Can you work these out from the model? Positions are in its coordinate system, mm. A direction names the side the tool comes from. Round coordinates to 2 decimals unless told otherwise and drop trailing zeros. Order: outer loops, then holes, each group sorted by start corner. A loop starts at its lowest first (then second) coordinate and runs counter-clockwise, first axis right, second up.
Q1. If I drill on line 1 (Y direction, x = 13.75, z = 0.55); line 2 (Y direction, x = -9, z = 2.55); line 3 (Y direction, x = 13.75, z = 0.5), over which ranges is the centre line in solid material (lowest first)?
Q2. For faces 5 (the face through (-11.61, 17.9, 2.36)), 6 (the face through (-18.05, -3.64, 3.43)), 7 (the face through (13.3, 23, 0.5)), 8 (the face through (16, 17, 2)), which set-ups out of +Z, -Z, +X, -X, +Y, -Y let a thin tool reach every point of the face, with its end or its side?
Q3. If we section it at A-A (y = -17.5): Please give me the cut outline in (x, z) (3 decimals), plus the area to 3 significant figures.
Q4. Will these pins go through, and if not, where does the flat tip stop? P1, Ø3, axis at x = 11.5, y = 13, coming from the -Z side; P2, Ø1.9, axis at y = 22, z = 2, coming from the -X side; P3, Ø3, axis at x = -14.5, y = 20, coming from the +Z side; P4, Ø1.4, axis at x = 15.5, z = 2, coming from the +Y side.
Q5. We'd pull the mould along Y, two halves only. Please class faces 1 (the face through (0, 1, 0)), 2 (the face through (-13.2, 23, 0.5)), 3 (the face through (12.64, 21.01, 0.49)), 4 (the face through (-14.86, 21.01, 0.49)): pulls with the +Y half, pulls with the -Y half, needs draft (parallel to the pull), parting line crosses it, or undercut.
from build123d import *

# Parameters (mm, degrees)
RESSALTO_EXTRUS_O1_DEPTH = 3.75
ESBO_O1_3_R              = 1.5
RESSALTO_EXTRUS_O2_DEPTH = 1
CORTE_EXTRUS_O1_DEPTH    = 46.225131288
CORTE_EXTRUS_O2_DEPTH    = 54.531532763


with BuildPart() as part:
    # Esbo_o1 → Ressalto-extrus_o1 (new body)
    with BuildSketch(Plane.XY):
        with BuildLine():
            Line((-10.75, 25), (-10.75, 20))
            ThreePointArc((-10.75, 20), (-11.628679656, 17.878679656), (-13.75, 17))
            Line((-13.75, 17), (-18.75, 17))
            Line((-18.75, 17), (-18.75, -25))
            Line((-18.75, -25), (18.75, -25))
            Line((18.75, -25), (18.75, 17))
            Line((18.75, 17), (13.75, 17))
            ThreePointArc((13.75, 17), (11.628679656, 17.878679656), (10.75, 20))
            Line((10.75, 20), (10.75, 25))
            Line((10.75, 25), (-10.75, 25))
        make_face()
    extrude(amount=RESSALTO_EXTRUS_O1_DEPTH)

    # Esbo_o1_3 → Ressalto-extrus_o2 (add)
    # profile 1 of 2: a face of its own
    with BuildSketch(Plane.XY):
        with BuildLine():
            Line((15.75, 23), (10.75, 23))
            Line((10.75, 23), (10.75, 20))
            ThreePointArc((10.75, 20), (11.628679656, 17.878679656), (13.75, 17))
            Line((13.75, 17), (18.75, 17))
            Line((18.75, 17), (18.75, 20))
            ThreePointArc((18.75, 20), (17.871320344, 22.121320344), (15.75, 23))
        make_face()
        with Locations((13.75, 20)):
            Circle(ESBO_O1_3_R, mode=Mode.SUBTRACT)
    # profile 2 of 2: a face of its own
    with BuildSketch(Plane.XY):
        with BuildLine():
            Line((-10.75, 20), (-10.75, 23))
            Line((-10.75, 23), (-15.75, 23))
            ThreePointArc((-15.75, 23), (-17.871320344, 22.121320344), (-18.75, 20))
            Line((-18.75, 20), (-18.75, 17))
            Line((-18.75, 17), (-13.75, 17))
            ThreePointArc((-13.75, 17), (-11.628679656, 17.878679656), (-10.75, 20))
        make_face()
        with Locations((-13.75, 20)):
            Circle(ESBO_O1_3_R, mode=Mode.SUBTRACT)
    extrude(amount=RESSALTO_EXTRUS_O2_DEPTH)

    # Esbo_o3 → Corte-extrus_o1 (cut, through all)
    with BuildSketch(Plane.ZY.offset(18.75)):
        with BuildLine():
            ThreePointArc((3.75, -23.257021896), (3.154999773, -24.49695337), (1.875, -25))
            Line((1.875, -25), (3.75, -25))
            Line((3.75, -25), (3.75, -23.257021896))
        make_face()
        with BuildLine():
            ThreePointArc((1.875, -25), (0.595000227, -24.49695337), (0, -23.257021896))
            Line((0, -23.257021896), (0, -25))
            Line((0, -25), (1.875, -25))
        make_face()
    extrude(amount=-CORTE_EXTRUS_O1_DEPTH, mode=Mode.SUBTRACT)

    # Esbo_o4 → Corte-extrus_o2 (cut, through all)
    with BuildSketch(Plane(origin=(0, 25, 0), x_dir=(1, 0, 0), z_dir=(0, 1, 0))):
        with BuildLine():
            Line((17, -4.75), (-17, -4.75))
            ThreePointArc((-17, -4.75), (-19.875, -1.875), (-17, 1))
            Line((-17, 1), (17, 1))
            ThreePointArc((17, 1), (19.875, -1.875), (17, -4.75))
        make_face()
        with BuildLine():
            Line((17, -3.75), (-17, -3.75))
            ThreePointArc((-17, -3.75), (-18.875, -1.875), (-17, 0))
            Line((-17, 0), (17, 0))
            ThreePointArc((17, 0), (18.875, -1.875), (17, -3.75))
        make_face(mode=Mode.SUBTRACT)
    extrude(amount=-CORTE_EXTRUS_O2_DEPTH, mode=Mode.SUBTRACT)


solid = part.part
Solution:
1. line 1: y = -24.45 to 18.5, 21.5 to 23
1. line 2: y = -24.87 to 25
1. line 3: y = -24.4 to 18.5, 21.5 to 23
2. face 5: +Z, -X, +Y
2. face 6: +Z, -X, +Y, -Y
2. face 7: +Z, -Z, +X, +Y
2. face 8: +Z, +X, +Y
3. outline: (-18.75, 1.202) arc R1.875 ccw to (-17, 0) - (17, 0) arc R1.875 ccw to (18.75, 1.202) - (18.75, 2.548) arc R1.875 ccw to (17, 3.75) - (-17, 3.75) arc R1.875 ccw to (-18.75, 2.548) - close
3. area: 138 mm2
4. P1: stops at z = 0
4. P2: stops at x = -10.75
4. P3: stops at z = 1
4. P4: stops at y = 17
5. face 1: needs draft
5. face 2: pulls with the +Y half
5. face 3: undercut
5. face 4: undercut
